Input: part model. Units: mm. Frame: model coordinates. Face numbers are marked on the shaded views. Coordinates: 2 decimals unless noted, no trailing zeros. Loops run counter-clockwise (first coordinate to the right, second up) from the corner with the lowest first, then second, coordinate; pieces in that order, holes last. Notation, with made-up numbers: (78, 54.5) -> (126, 54.5) arc R28 cw to (126, 87.5) -> close; hole circle Ø4 at (49.5, 12.5). An arc over 180 degrees is marked (long way). Put each result on its own line as item: value. Start each with the question number.
1) Material intervals for L1, parallel to Y at x = 0, z = 55.5; L2, parallel to X at y = 1.25, z = 77.5; L3, parallel to X at y = -4.25, z = 9.5, sorted ascending.
2) Cut plane A-A (y = 0). Return the cut outline in (x, z), plus the area to 3 significant figures.
3) Cut plane C-C (z = 21.5). Return the cut outline in (x, y), plus the area to 3 significant figures.
4) Pull-direction query (X, two-part tool) for the marked faces 1, 2 and 3; classes: pulls with the +X half, pulls with the -X half, needs draft (parallel to the pull), parting line crosses it, or undercut.
5) Contact query for flat-ended pins moving along their axis: P1, Ø3, axis at x = 3, z = 33.5, coming from the -Y side; P2, Ø1.5, axis at y = -3.5, z = 36.5, coming from the -X side; P3, Ø1.5, axis at y = 8, z = 41.5, coming from the -X side. Output: stop coordinate, or through.
from build123d import *

# Parameters (mm, degrees)
SKETCH_1_R      = 15
SKETCH_1_R_2    = 7
EXTRUDE_1_DEPTH = 80
CHAMFER_1_SIZE  = 1
CHAMFER_2_SIZE  = 2


with BuildPart() as part:
    # Эскиз1 → Бобышка-Вытянуть1 (new body)
    with BuildSketch(Plane.XY):
        Circle(SKETCH_1_R)
        Circle(SKETCH_1_R_2, mode=Mode.SUBTRACT)
    extrude(amount=EXTRUDE_1_DEPTH)

    # Фаска1
    chamfer_1_edges = [part.edges().sort_by_distance(p)[0] for p in [
        (-7, 0, 0),
        (-7, 0, 80),
    ]]
    chamfer(chamfer_1_edges, length=CHAMFER_1_SIZE)

    # Фаска2
    chamfer_2_edges = [part.edges().sort_by_distance(p)[0] for p in [
        (-15, 0, 0),
        (-15, 0, 80),
    ]]
    chamfer(chamfer_2_edges, length=CHAMFER_2_SIZE)


solid = part.part
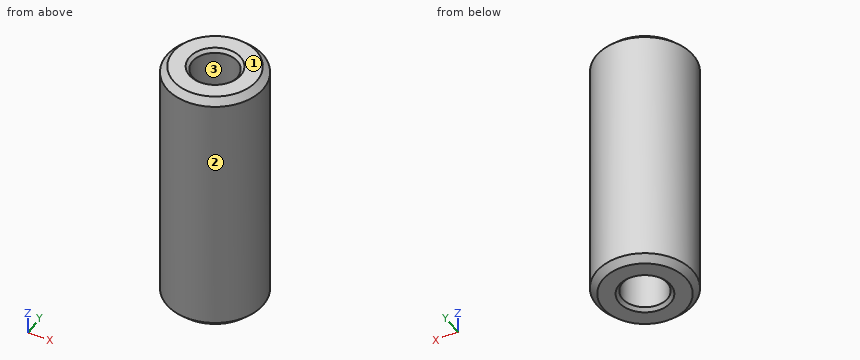
Results found:
1. L1: y = -15 to -7, 7 to 15
1. L2: x = -14.95 to -6.89, 6.89 to 14.95
1. L3: x = -14.39 to -5.56, 5.56 to 14.39
2. outline: (-15, 2) -> (-13, 0) -> (-8, 0) -> (-7, 1) -> (-7, 79) -> (-8, 80) -> (-13, 80) -> (-15, 78) -> close; (7, 1) -> (8, 0) -> (13, 0) -> (15, 2) -> (15, 78) -> (13, 80) -> (8, 80) -> (7, 79) -> close
2. area: 1,270 mm2
3. outline: circle Ø30 at (0, 0); hole circle Ø14 at (0, 0)
3. area: 553 mm2
4. face 1: needs draft
4. face 2: parting line crosses it
4. face 3: undercut
5. P1: stops at y = -14.92
5. P2: stops at x = -14.75
5. P3: stops at x = -13.13
